Check sheet for the drawn part. Datum: minimum x, y, z corner. Units: mm. A direction names the side the tool comes from. Coordinates: 2 decimals unless noted, no trailing zeros. Order: outer loops, then holes, each group sorted by start corner. A loop starts at its lowest first (then second) coordinate and runs counter-clockwise, first axis right, second up. Notation, with made-up numbers: (38.25, 42) - (72.25, 42) arc R4 cw to (72.25, 48) - close; hole circle Ø8 at (-21.5, 53.5). An arc over 180 degrees is marked (long way). Put each result on its own line as item: value.
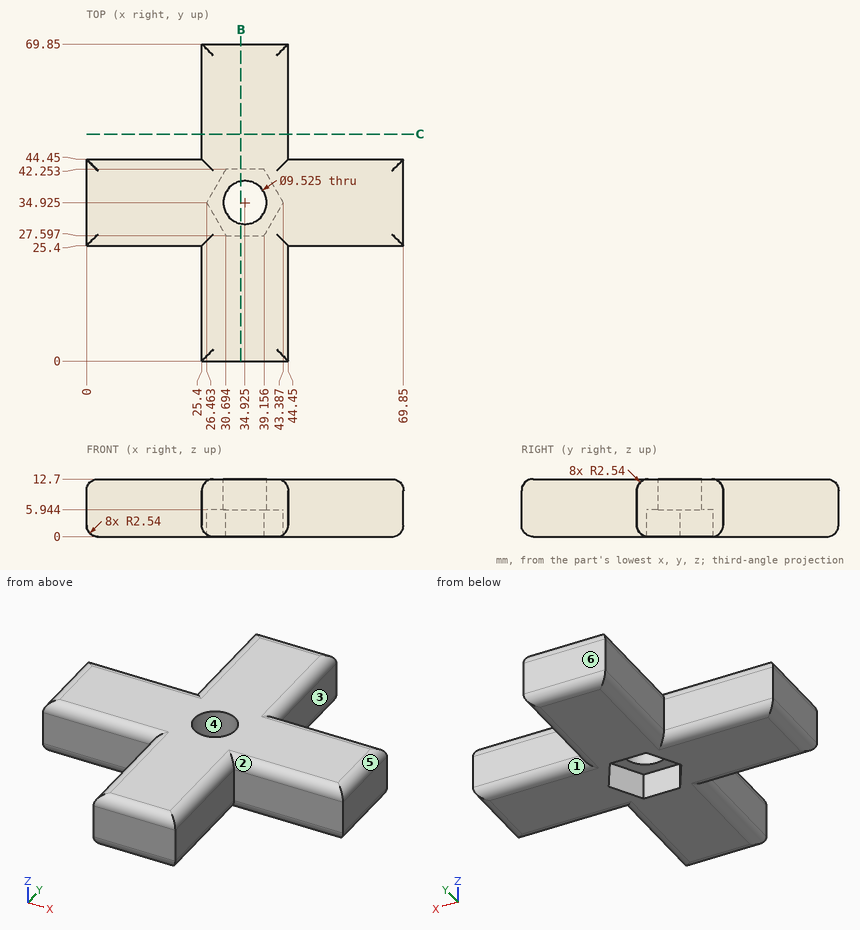
Q1. Depth check by flat-ended pin: pin 1 Ø4 at (x, z) = (61, 6.5) entering from -Y; pin 2 Ø4 at (y, z) = (12.5, 6.5) entering from -X; pin 3 Ø4 at (y, z) = (18, 5) entering from +X. Enter the tip coordinate at first touch or a pass-through.
Answer block:
pin 1: stops at y = 25.4
pin 2: stops at x = 25.4
pin 3: stops at x = 44.45
Q2. Access from +Z, -Z, +X, -X, +Y, -Y to the whole of each face (thin tool, end or side, straight path). Record for the marked faces 1, 2 and 3.
Answer block:
face 1: -Z, +X, +Y
face 2: +Z, +X, -Y
face 3: +Z, -Z, +X, +Y
Q3. Section check C-C on y = 50. Record the boundary of the cut face in (x, z).
Answer block:
outline: (25.4, 2.54) arc R2.54 ccw to (27.94, 0) - (41.91, 0) arc R2.54 ccw to (44.45, 2.54) - (44.45, 10.16) arc R2.54 ccw to (41.91, 12.7) - (27.94, 12.7) arc R2.54 ccw to (25.4, 10.16) - close
Q4. Thickness scan on L1, parallel to Y at x = 57, z = 6.5; L2, parallel to Y at x = 66.5, z = 12. Record the ranges inside material, lowest first. Write a range as [from, to].
Answer block:
L1: y = [25.4, 44.45]
L2: y = [26.19, 43.66]
Q5. Draft check along Y on the marked faces 4, 5 and 6. Enter one of: pulls with the +Y half, pulls with the -Y half, needs draft (parallel to the pull), parting line crosses it, or undercut.
Answer block:
face 4: undercut
face 5: needs draft
face 6: pulls with the +Y half
Q6. Section check B-B on x = 34. Record the boundary of the cut face in (y, z), then the cut area to 3 significant figures.
Answer block:
outline: (0, 2.54) arc R2.54 ccw to (2.54, 0) - (27.6, 0) - (27.6, 5.94) - (30.25, 5.94) - (30.25, 12.7) - (2.54, 12.7) arc R2.54 ccw to (0, 10.16) - close; (39.6, 5.94) - (42.25, 5.94) - (42.25, 0) - (67.31, 0) arc R2.54 ccw to (69.85, 2.54) - (69.85, 10.16) arc R2.54 ccw to (67.31, 12.7) - (39.6, 12.7) - close
area: 731 mm^2
